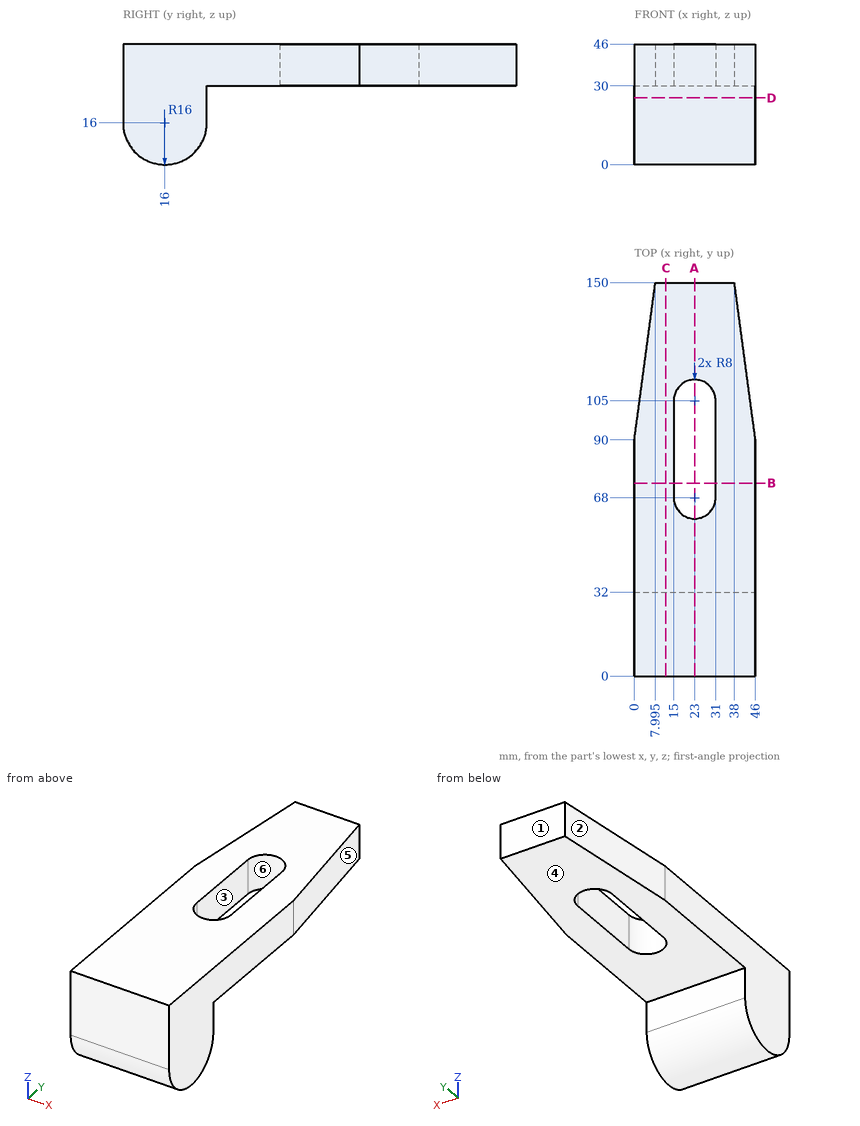
Part print with two shaded views. Sizes in mm from the minimum x, y, z corner. A direction names the side the tool comes from. Coordinates: 2 decimals unless noted, no trailing zeros. Loops run counter-clockwise (first coordinate to the right, second up) from the corner with the lowest first, then second, coordinate; pieces in that order, holes last. Notation, with made-up numbers: (-5.75, 11) -> (31.25, 11) arc R13 ccw to (31.25, 19) -> close; hole circle Ø10 at (24, 9.25). An arc over 180 degrees is marked (long way). Answer as a JSON object with one key per item and string values.
Q1. Cut at C-C (x = 12). List the corners of the cut face in (y, z), and give its area (3 significant figures).
Report:
{"outline": "(0, 16) arc R16 ccw to (32, 16) -> (32, 30) -> (150, 30) -> (150, 46) -> (0, 46) -> close", "area": "3,250 mm2"}
Q2. Cut at B-B (y = 73.5). List the corners of the cut face in (x, z).
Report:
{"outline": "(0, 30) -> (15, 30) -> (15, 46) -> (0, 46) -> close; (31, 30) -> (46, 30) -> (46, 46) -> (31, 46) -> close"}
Q3. Cut at A-A (x = 23). List the corners of the cut face in (y, z), and give its area (3 significant figures).
Report:
{"outline": "(0, 16) arc R16 ccw to (32, 16) -> (32, 30) -> (60, 30) -> (60, 46) -> (0, 46) -> close; (113, 30) -> (150, 30) -> (150, 46) -> (113, 46) -> close", "area": "2,400 mm2"}
Q4. Probe probe 1 along X at (y, z) = (72.5, 31.5); probe 2 along Z at (x, y) = (42.5, 75); probe 3 along Z at (x, y) = (15, 15). List the from-to ranges inside material, lowest first.
Report:
{"probe 1": "x = 0 to 15, 31 to 46", "probe 2": "z = 30 to 46", "probe 3": "z = 0.03 to 46"}
Q5. Cut at D-D (z = 25.5). List the corners of the cut face in (x, y), and give its area (3 significant figures).
Report:
{"outline": "(0, 0) -> (46, 0) -> (46, 32) -> (0, 32) -> close", "area": "1,470 mm2"}
Q6. 3-axis set-ups, long thin cutter, end or side, ignore diameter. For the marked faces 4, 5 and 6: which of +Z, -Z, +X, -X, +Y, -Y reach the whole face in a straight line?
Report:
{"face 4": "-Z, +X, -X, +Y", "face 5": "+Z, -Z, +X, +Y", "face 6": "+Z, -Z"}
Q7. Pull direction X, two halves, no side cores. Call the marked faces 1, 2 and 3: released by +X, released by -X, zero draft, split by the parting line, or undercut.
Report:
{"face 1": "zero draft", "face 2": "released by -X", "face 3": "undercut"}
Q8. Flat gauge pins, fed straight in: P1, Ø6, axis at y = 128.5, z = 37, coming from the +X side; P2, Ø10, axis at y = 69, z = 22, coming from the -X side; P3, Ø11, axis at x = 28.5, z = 24, coming from the +Y side; P4, Ø2, axis at x = 36, y = 45.5, coming from the -Z side. Where does each tip first touch, or does it go through?
Report:
{"P1": "stops at x = 41.27", "P2": "passes through", "P3": "stops at y = 32", "P4": "stops at z = 30"}
